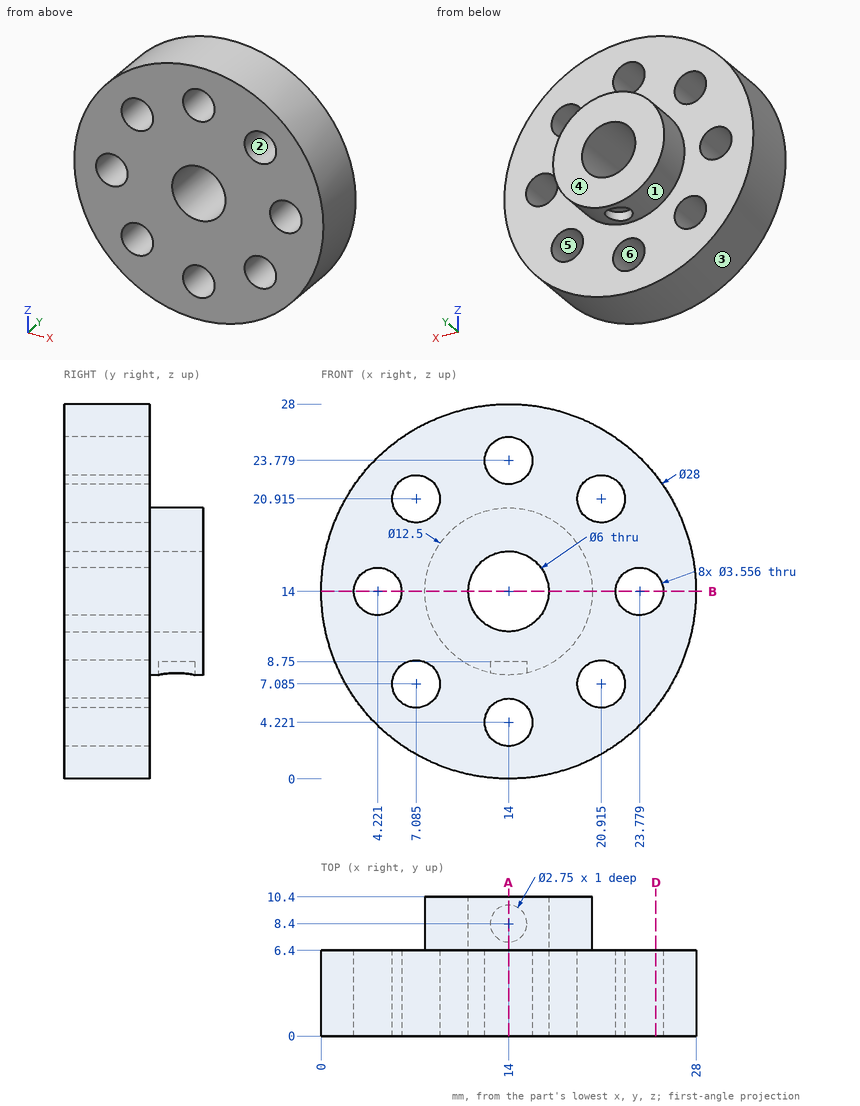
Job drawing, mm, ordinate dimensions from the low corner. One solid piece. A direction names the side the tool comes from. Coordinates: 2 decimals unless noted, no trailing zeros. Order: outer loops, then holes, each group sorted by start corner. A loop starts at its lowest first (then second) coordinate and runs counter-clockwise, first axis right, second up. Notation, with made-up numbers: M -28.5,-37.75 L -20.5,-37.75 A29 ccw -20.5,-13.75 Z; hole C -0.75,-0.75 d10. An arc over 180 degrees is marked long. Return JSON: item names as keys, results as strings.
1. Pull direction Z, two halves, no side cores. Call the marked faces 3, 4, 5 and 6: +Z half, -Z half, draft (parallel to the pull), parting line (faces both ways), or undercut.
Ans:
{"face 3": "parting line", "face 4": "draft", "face 5": "undercut", "face 6": "undercut"}
2. Saw through at D-D (x = 25). Give the cut face in (y, z), and give its area (3 significant figures).
Ans:
{"outline": "M 0,5.34 L 6.4,5.34 L 6.4,12.71 L 0,12.71 Z; M 0,15.29 L 6.4,15.29 L 6.4,22.66 L 0,22.66 Z", "area": "94.3 mm^2"}
3. Saw through at A-A (x = 14). Give the cut face in (y, z) (3 decimals).
Ans:
{"outline": "M 0,0 L 6.4,0 L 6.4,2.443 L 0,2.443 Z; M 0,5.999 L 6.4,5.999 L 6.4,7.75 L 7.025,7.75 L 7.025,8.75 L 9.775,8.75 L 9.775,7.75 L 10.4,7.75 L 10.4,11 L 0,11 Z; M 0,17 L 10.4,17 L 10.4,20.25 L 6.4,20.25 L 6.4,22.001 L 0,22.001 Z; M 0,25.557 L 6.4,25.557 L 6.4,28 L 0,28 Z"}
4. Saw through at B-B (z = 14). Give the cut face in (x, y).
Ans:
{"outline": "M 0,0 L 2.44,0 L 2.44,6.4 L 0,6.4 Z; M 6,0 L 11,0 L 11,10.4 L 7.75,10.4 L 7.75,6.4 L 6,6.4 Z; M 17,0 L 22,0 L 22,6.4 L 20.25,6.4 L 20.25,10.4 L 17,10.4 Z; M 25.56,0 L 28,0 L 28,6.4 L 25.56,6.4 Z"}
5. Drill centre lines: probe 1 along Z at (x, y) = (7.75, 2) (1 decimal); probe 2 along Z at (x, y) = (6.5, 2.5) (1 decimal); probe 3 along Y at (x, z) = (16.5, 2.25). Where is each one in solid material? Low to high.
Ans:
{"probe 1": "1.5 to 5.4, 8.7 to 19.3, 22.6 to 26.5", "probe 2": "2.2 to 5.4, 8.8 to 19.2, 22.6 to 25.8", "probe 3": "0 to 6.4"}
6. Flat gauge pins, fed straight in: pin 1 (1 mm diameter, centred on y = 7.5, z = 10, fed in from +X); pin 2 (1 mm diameter, centred on y = 1.5, z = 25, fed in from -X); pin 3 (5 mm diameter, centred on y = 5.5, z = 6.5, fed in from -X); pin 4 (3 mm diameter, centred on x = 7.09, z = 20.91, fed in from +Y). Where does each tip first touch, or does it go through?
Ans:
{"pin 1": "x = 19.18", "pin 2": "x = 4.74", "pin 3": "x = 0.92", "pin 4": "through"}
7. Tool access for the marked faces 1 and 2: list every direction of +Z, -Z, +X, -X, +Y, -Y with a clear straight run to the whole face (end or side of a thin tool).
Ans:
{"face 1": "+Y", "face 2": "+Y, -Y"}
